```python
from build123d import *

# Parameters (mm, degrees)
ESQUISSE1_W             = 22
ESQUISSE1_H             = 56.5
ESQUISSE2_R             = 17
ENL_V_MAT_EXTRU_1_DEPTH = 93.420235879


with BuildPart() as part:
    # Esquisse1 → Révolution1 (revolve)
    with BuildSketch(Plane.XY, mode=Mode.PRIVATE) as r_volution1_sk:
        with Locations((-11, 28.25)):
            Rectangle(ESQUISSE1_W, ESQUISSE1_H)
        Polygon((0, 56.5), (0, 0), (3, 0), (3, 57.5), (0, 62.5), align=None)
        Polygon((-24, 0), (-22, 0), (-22, 56.5), (-22, 62.5), (-24, 62.5), align=None)
    revolve(r_volution1_sk.sketch.rotate(Axis((-24, 0, 0), (1, 0, 0)), 180), axis=Axis((-24, 0, 0), (1, 0, 0)))

    # Esquisse2 → Enlèv. mat.-Extru.1 (cut, through all)
    with BuildSketch(Plane.ZY.offset(24)):
        with Locations(Location((0, 0, 0), (0, 0, 270))):
            Circle(ESQUISSE2_R)
    extrude(amount=-ENL_V_MAT_EXTRU_1_DEPTH, mode=Mode.SUBTRACT)


solid = part.part
```
Part model, mm, in its own coordinate system. A direction names the side the tool comes from. Round coordinates to 2 decimals unless told otherwise and drop trailing zeros. Order: outer loops, then holes, each group sorted by start corner. A loop starts at its lowest first (then second) coordinate and runs counter-clockwise, first axis right, second up. Notation, with made-up numbers: M 31,22.5 L 61,22.5 A24 ccw 61,37.5 Z; hole C 61.25,-16.75 d9. An arc over 180 degrees is marked long. Answer in a Markdown table with one row per item. Add a question column.
Q1. 3-axis set-ups, long thin cutter, end or side, ignore diameter. For faces 1 (the face through (3, 12, -14)), 2 (the face through (0, 47, 32)): which of +Z, -Z, +X, -X, +Y, -Y reach the whole face in a straight line?
Q2. Mould opens along Z. For faces 3 (the face through (-10.689, 2.213, 16.855)), 4 (the face through (-23.01, 62.44, -2.75)), 5 (the face through (-22, -47, 32)) say: +Z half, -Z half, draft (parallel to the pull), parting line (faces both ways), or undercut.
Q3. Wall check: L1, parallel to Z at x = -6.25, y = 0; L2, parallel to Z at x = -15.75, y = 9; L3, parallel to X at y = -17.5, z = -55.5. Give the ranges that are in metal, low to high. Write a range as from..to.
Q4. Cut at C-C on x = -2.75. Give the cut face in (y, z).
Q5. Pin check, flat tips, straight feed: pin 1 (2 mm diameter, centred on x = -0.5, y = -44, fed in from -Z); pin 2 (2 mm diameter, centred on x = -4, z = -47.5, fed in from +Y); pin 3 (4 mm diameter, centred on x = -8.5, y = 20, fed in from +Z). Stop position of each tip, or through.
Q6. Cut at A-A on z = 0. Give the cut face in (x, y), and give its area (3 significant figures).
Established:
| question | item | result |
|---|---|---|
| 1 | face 1 | +Z, -Z, +X, +Y, -Y |
| 1 | face 2 | none |
| 2 | face 3 | undercut |
| 2 | face 4 | parting line |
| 2 | face 5 | draft |
| 3 | L1 | z = -56.5..-17, 17..56.5 |
| 3 | L2 | z = -55.78..-14.42, 14.42..55.78 |
| 3 | L3 | x = -24..-22, 0..2.58 |
| 4 | outline | C 0,0 d113; hole C 0,0 d34 |
| 5 | pin 1 | stops at z = -45.23 |
| 5 | pin 2 | stops at y = 32.09 |
| 5 | pin 3 | stops at z = 53.56 |
| 6 | outline | M -24,-62.5 L -22,-62.5 L -22,-56.5 L 0,-56.5 L 0,-62.5 L 3,-57.5 L 3,-17 L -24,-17 Z; M -24,17 L 3,17 L 3,57.5 L 0,62.5 L 0,56.5 L -22,56.5 L -22,62.5 L -24,62.5 Z |
| 6 | area | 2,180 mm2 |
